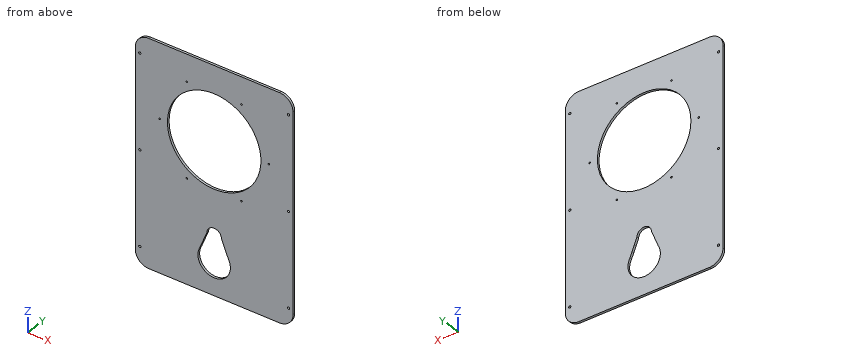
Autodesk Inventor part; units mm, degrees
ref_plane "YZ Plane" through (0, 0, 0) normal (1, 0, 0) x (0, 1, 0)
ref_plane "XZ Plane" through (0, 0, 0) normal (0, 1, 0) x (-1, 0, 0)
ref_plane "XY Plane" through (0, 0, 0) normal (0, 0, 1) x (1, 0, 0)
sketch "스케치1" plane through (0, 0, 0) normal (0, 1, 0) x (-1, 0, 0)
  line L0 (145, 250) -> (-145, 250)
  line L1 (-175, 220) -> (-175, -220)
  line L2 (-145, -250) -> (145, -250)
  line L3 (175, -220) -> (175, 220)
  line L4 (175, 250) -> (-175, -250) construction
  line L5 (-175, 250) -> (175, -250) construction
  circle A0 centre (0, -175) radius 36
  arc A1 (145, -250) -> (175, -220) centre (145, -220) ccw
  arc A2 (-175, -220) -> (-145, -250) centre (-145, -220) ccw
  arc A3 (-145, 250) -> (-175, 220) centre (-145, 220) ccw
  arc A4 (175, 220) -> (145, 250) centre (145, 220) ccw
  circle A5 centre (0, 85) radius 103.75
  point P0 (0, 0)
  dimension "d0" = 350
  dimension "d1" = 500
  dimension "d2" = 72
  dimension "d3" = 30
  dimension "d4" = 75
  dimension "d5" = 207.5
  dimension "d7" = 165
extrude "돌출1" add sketch "스케치1" along normal blind 5
sketch "스케치2" plane through (0, 0, 0) normal (0, -1, 0) x (1, 0, 0)
  line L0 (-145, 250) -> (145, 250)
  line L1 (-175, -220) -> (-175, 220)
  line L2 (145, -250) -> (-145, -250)
  line L3 (175, 220) -> (175, -220)
  circle A0 centre (165, 210) radius 2.5
  line L4 (0, 250) -> (0, -250) construction
  line L5 (-175, 0) -> (175, 0) construction
  circle A1 centre (165, -210) radius 2.5
  circle A2 centre (165, 0) radius 2.5
  circle A3 centre (-165, 210) radius 2.5
  circle A4 centre (-165, -210) radius 2.5
  circle A5 centre (-165, 0) radius 2.5
  point P0 (0, 0)
  dimension "d11" = 5
  dimension "d12" = 40
  dimension "d13" = 10
  dimension "d14" = 5
  dimension "d15" = 10
extrude "돌출2" cut sketch "스케치2" against normal through all
sketch "스케치3" plane through (0, 5, 0) normal (0, 1, 0) x (1, 0, 0)
  circle A0 centre (0, 175) radius 36
  circle A1 centre (0, 175) radius 33.15
  line L0 (0, 175) -> (0, 119.3)
  circle A2 centre (-55.0502, 292.3468) radius 36
  line L1 (26.9254, 146.1085) -> (31.6003, 157.7541)
  line L2 (15.9944, 118.8781) -> (21.8404, 133.441)
  arc A3 (-15.9945, 118.88) -> (15.9944, 118.8781) centre (0, 119.3) ccw
  line L3 (-20.7535, 130.7351) -> (-15.9945, 118.88)
  line L4 (-31.5976, 157.7491) -> (-25.8385, 143.4026)
  circle A4 centre (-55.0502, 292.3468) radius 36
  circle A5 centre (-55.0502, 292.3468) radius 36
  line L5 (-20.7535, 130.7351) -> (-25.8385, 143.4026)
  line L6 (21.8404, 133.441) -> (26.9254, 146.1085)
  arc A6 (-13.9206, 113.7129) -> (13.92, 113.7112) centre (0, 119.3) ccw construction
  line L7 (13.92, 113.7112) -> (15.9944, 118.8781) construction
  line L8 (-13.9206, 113.7129) -> (-15.9945, 118.88) construction
  point P0 (0, 0)
  dimension "d18" = 12.7747
  dimension "d19" = 13.65
  dimension "d21" = 16
  dimension "d22" = 15
  dimension "d23" = 176.985
  dimension "d24" = 136.256
  dimension "d25" = 5.5678
  dimension "d26" = 5.5678
  dimension "d27" = 55.7
  dimension "d28" = 15.6925
  dimension "d29" = 13.65
  dimension "d31" = 43.744
  dimension "d32" = 43.744
  dimension "d33" = 43.744
  dimension "d34" = 12.5489
  dimension "d35" = 15.4593
extrude "돌출3" cut sketch "스케치3" against normal blind 10 contours A0 L1 L6 L2 A3 L3 L5 L4
sketch "스케치4" plane through (0, 5, 0) normal (0, 1, 0) x (1, 0, 0)
  circle A0 centre (0, -85) radius 103.75
  circle A1 centre (-0.0796, -85.0052) radius 104.02
  line L0 (-0.0796, -85.0052) -> (-121.1411, -85.0052) construction
  line L1 (-0.0796, -85.0052) -> (120.9819, -85.0052) construction
  circle A2 centre (-121.1411, -85.0052) radius 1.8
  circle A3 centre (-60.566, -189.9139) radius 1.8
  circle A4 centre (60.5751, -189.9087) radius 1.8
  circle A5 centre (121.1411, -84.9948) radius 1.8
  circle A6 centre (60.566, 19.9139) radius 1.8
  circle A7 centre (-60.5751, 19.9087) radius 1.8
  point P0 (0, 0)
  dimension "d38" = 121.0615
  dimension "d39" = 180
  dimension "d40" = 3.6
  dimension "d43" = 360
extrude "돌출4" cut sketch "스케치4" against normal blind 10 contours A2 | A3 | A4 | A5 | A6 | A7
properties part number "부품8"
Could you check a few things on this model? Use its own coordinates, in mm. Give positions to 0.01 mm unless a question says otherwise; leave off trailing zeros. Order: outer loops, then holes, each group sorted by start corner. A loop starts at its lowest first (then second) coordinate and runs counter-clockwise, first axis right, second up.
Q1. Suppose I cut it at B-B, the plane z = -175. Write out the boundary of the cut face in (x, y).
Q2. Suppose I cut it at D-D, the plane y = 2.05. Count the separate pieces of the cut face and the enclosed holes in it, and give its area (3 significant figures).
Q3. I'm going to push a flat-ended pin straight in: P1, Ø2, axis at x = -121.14, z = 85.01, coming from the +Y side. Where does the tip first touch, or does it pass through?
Q4. Suppose I cut it at C-C, the plane x = 72.5. Write out the boundary of the cut face in (y, z).
Q5. If I drill on line 1 along X through (y, z) = (1.75, 210); line 2 along X through (y, z) = (3.25, -175); line 3 along X through (y, z) = (4.2, 2), over which ranges is the centre line in solid material (lowest first)?
Q6. Suppose I cut it at A-A, the plane x = 0. Write out the boundary of the cut face in (y, z).
Solution:
1. outline: (-175, 0) - (-36, 0) - (-36, 5) - (-175, 5) - close; (36, 0) - (175, 0) - (175, 5) - (36, 5) - close
2. separate pieces: 1
2. enclosed holes: 14
2. area: 135,000 mm2
3. P1: passes through
4. outline: (0, -250) - (5, -250) - (5, 10.79) - (0, 10.79) - close; (0, 159.21) - (5, 159.21) - (5, 250) - (0, 250) - close
5. line 1: x = -175 to -167.5, -162.5 to 162.5, 167.5 to 175
5. line 2: x = -175 to -36, 36 to 175
5. line 3: x = -175 to -166.5, -163.5 to -62.25, 62.25 to 163.5, 166.5 to 175
6. outline: (0, -250) - (5, -250) - (5, -211) - (0, -211) - close; (0, -103.3) - (5, -103.3) - (5, -18.75) - (0, -18.75) - close; (0, 188.75) - (5, 188.75) - (5, 250) - (0, 250) - close
